Autodesk Fusion 360 part; units mm, degrees
sketch "Esboço1" plane through (0, 0, 0) normal (0, 0, 1) x (1, 0, 0)
  circle A0 centre (0, 0) radius 19
  circle A1 centre (0, 0) radius 20.5
  dimension "d1" = 38
  dimension "d2" = 41
extrude "Extrusão1" add sketch "Esboço1" along normal blind 60
extrude "Extrusão2" add sketch "Esboço1" along normal blind 3 contours A0
sketch "Esboço2" plane through (0, 0, 0) normal (0, 0, 1) x (1, 0, 0)
  circle A0 centre (15, 0) radius 2
  circle A1 centre (7.5, 12.9904) radius 2
  circle A2 centre (-7.5, 12.9904) radius 2
  circle A3 centre (-15, 0) radius 2
  circle A4 centre (-7.5, -12.9904) radius 2
  circle A5 centre (7.5, -12.9904) radius 2
  dimension "d7" = 15
  dimension "d8" = 4
  dimension "d10" = 360
extrude "Extrusão3" cut sketch "Esboço2" along normal blind 11
sketch "Esboço3" plane through (0, 0, 0) normal (0, 0, 1) x (1, 0, 0)
  circle A0 centre (0, 7) radius 6.5
  dimension "d13" = 7
  dimension "d14" = 13
extrude "Extrusão4" cut sketch "Esboço3" along normal blind 24
sketch "Esboço4" plane through (0, 0, 0) normal (0, 0, 1) x (1, 0, 0)
  line L0 (-20.5, 0) -> (-25.5, 0)
  line L1 (-25.5, 0) -> (-25.5, 35.5)
  circle A0 centre (0, 0) radius 20.5
  line L2 (-20.5, 35.5) -> (-25.5, 35.5)
  line L3 (20.5, 0) -> (25.5, 0)
  line L4 (25.5, 0) -> (25.5, 35.5)
  line L5 (25.5, 35.5) -> (20.5, 35.5)
  line L6 (20.5, 35.5) -> (-20.5, 35.5)
  arc A1 (-25.5, 0) -> (25.5, 0) centre (0, 0) ccw
  dimension "d17" = 5
  dimension "d19" = 5
extrude "Extrusão9" add sketch "Esboço4" along normal mid plane 35 from surface at 30 contours L0 A0 L3 A1 | L0 L1 A0 L2 L3 L4 L5 L6
sketch "Esboço5" plane through (25.5, 0, 0) normal (1, 0, 0) x (0, 1, 0)
  line L0 (35.5, 12.5) -> (35.5, 47.5)
  line L1 (35.5, 47.5) -> (0, 47.5)
  line L2 (0, 47.5) -> (0, 12.5)
  line L3 (0, 12.5) -> (35.5, 12.5)
  line L4 (35.5, 37.5) -> (20.5, 37.5)
  line L5 (20.5, 37.5) -> (20.5, 22.5)
  line L6 (20.5, 22.5) -> (35.5, 22.5)
  line L7 (35.5, 37.5) -> (35.5, 22.5)
  dimension "d35" = 15
extrude "Extrusão10" cut sketch "Esboço5" against normal blind 59 contours L0 L4 L5 L6 L7
sketch "Esboço6" plane through (0, 0, 47.5) normal (0, 0, 1) x (-1, 0, 0)
  circle A0 centre (0, 0) radius 20.5
  arc A1 (25.5, 0) -> (-25.5, 0) centre (0, 0) ccw
  line L0 (-25.5, 0) -> (-25.5, -35.5)
  line L1 (-25.5, -35.5) -> (25.5, -35.5)
  line L2 (25.5, -35.5) -> (25.5, 0)
  circle A2 centre (-18.5, -28) radius 2
  circle A3 centre (18.5, -28) radius 2
  dimension "d42" = 4
  dimension "d43" = 4
extrude "Extrusão11" cut sketch "Esboço6" against normal blind 43 contours A2 | A3
sketch "Esboço7" plane through (0, 0, 47.5) normal (0, 0, 1) x (-1, 0, 0)
  circle A0 centre (-18.5, -28) radius 2
  circle A1 centre (18.5, -28) radius 2
  circle A2 centre (0, 0) radius 20.5
  arc A3 (25.5, 0) -> (-25.5, 0) centre (0, 0) ccw
  line L0 (-25.5, 0) -> (-25.5, -35.5)
  line L1 (-25.5, -35.5) -> (25.5, -35.5)
  line L2 (25.5, -35.5) -> (25.5, 0)
  line L3 (-15.5, -26.2679) -> (-18.5, -24.5359)
  line L4 (-18.5, -24.5359) -> (-21.5, -26.2679)
  line L5 (-21.5, -26.2679) -> (-21.5, -29.7321)
  line L6 (-21.5, -29.7321) -> (-18.5, -31.4641)
  line L7 (-18.5, -31.4641) -> (-15.5, -29.7321)
  line L8 (-15.5, -29.7321) -> (-15.5, -26.2679)
  line L9 (21.4679, -29.7865) -> (21.5311, -26.3229)
  line L10 (21.5311, -26.3229) -> (18.5632, -24.5365)
  line L11 (18.5632, -24.5365) -> (15.5321, -26.2135)
  line L12 (15.5321, -26.2135) -> (15.4689, -29.6771)
  line L13 (15.4689, -29.6771) -> (18.4368, -31.4635)
  line L14 (18.4368, -31.4635) -> (21.4679, -29.7865)
  point P0 (-18.5, -28)
  point P1 (18.5, -28)
  dimension "d46" = 3
  dimension "d47" = 3
extrude "Extrusão12" cut sketch "Esboço7" against normal blind 2.8 contours L3 L4 L5 L6 L7 L8 | L9 L10 L11 L12 L13 L14
chamfer "Chanfro1" distance 1.5 distance2 1.5 2 edges at (20.3647, 28.7232, 12.5) (-16.6353, 28.7232, 12.5) measured on face at (0.5107, 26.232, 12.5) measured on face at (0.5107, 26.232, 12.5)
fillet "Arredondamento1" radius 1.5 10 edges at (-25.5, 17.75, 47.5) (0, -25.5, 47.5) (25.5, 17.75, 47.5) (25.5, 17.75, 12.5) (0, -25.5, 12.5) (-25.5, 17.75, 12.5) (0, 35.5, 47.5) (0, 35.5, 12.5) (-19.1127, -7.4131, 60) (-19.1127, -7.4131, 0)
fillet "Arredondamento2" radius 7 2 edges at (-19.1127, -7.4131, 47.5) (-19.1127, 7.4131, 12.5)
equation "d17 = d19"
equation "d46 = ( ( 5 / 2 ) * 1 mm ) + 0.5 * 1 mm"
equation "d47 = d46"
Work out the finished part from the listing and answer in its coordinate system (mm). A direction names the side the tool comes from. Give positions to 0.01 mm unless a question says otherwise; leave off trailing zeros. Write each loop counter-clockwise with the first axis right and the second up, starting at its lowest first coordinate (ties: lowest second). Pieces come first, ordered by that corner, then holes.
Q1. The part is cut by section B-B on x = -7.5. State how many separate pieces and enclosed holes the cut face has, and give its area (3 significant figures).
Answer:
separate pieces: 3
enclosed holes: 0
area: 843 mm2
Q2. Straight lines are drawn through the part: L1, parallel to Y at x = 7, z = 2; L2, parallel to Y at x = 0, z = 1.65; L3, parallel to Y at x = 0.5, z = 19. For each, find the intervals that lie inside material, in ascending order.
Answer:
L1: y = -19.27 to -14.93, -11.05 to 11.05, 14.93 to 19.27
L2: y = -20.5 to 0.5, 13.5 to 20.5
L3: y = -25.5 to -18.99, 18.99 to 35.5
Q3. A tool of negligible diameter and unlimited length cuts with its end or side. For faces 4 (the face through (20, 30.6, 46.1)), 5 (the face through (0, 35.5, 42)), 6 (the face through (-25.07, 17.5, 12.95)), 7 (the face through (-2.669, -20.326, 3.844)), from which of +Z, -Z, +X, -X, +Y, -Y can it reach the whole face along a straight path? Write none if from no direction.
Answer:
face 4: +Z
face 5: +Z, -Z, +X, -X, +Y
face 6: -Z, -X, +Y
face 7: -Z
Q4. The part is cut by section A-A on z = 26.5. Give the vertices of the cut face in (x, y), and give its area (3 significant figures).
Answer:
outline: (-25.5, 0) arc R25.5 ccw to (25.5, 0) - (25.5, 20.5) - (-25.5, 20.5) - close; hole circle Ø38 at (0, 0)
area: 933 mm2
Q5. Given pin 1 (4.5 mm diameter, centred on x = 18.5, y = 28, fed in from -Z); pin 2 (12 mm diameter, centred on x = 1, y = 26, fed in from +Z); pin 3 (5 mm diameter, centred on x = -17.5, y = 29, fed in from +Z), each flat-ended and moving along its own axis, determine where each tip first touches the part or whether it passes through.
Answer:
pin 1: stops at z = 13.75
pin 2: stops at z = 59.6
pin 3: stops at z = 47.5
Q6. For a pull along Z with two mould halves and no side action, classify faces 1 (the face through (0, 28, 22.5)), 2 (the face through (5.913, 14.207, 1.479)), 3 (the face through (0.36, 35.05, 12.93)) as released by +Z, released by -Z, zero draft, split by the parting line, or undercut.
Answer:
face 1: undercut
face 2: zero draft
face 3: released by -Z
